Can you work these out from the model? Positions are in its coordinate system, mm. A direction names the side the tool comes from. Round coordinates to 2 decimals unless told otherwise and drop trailing zeros. Loops run counter-clockwise (first coordinate to the right, second up) from the corner with the lowest first, then second, coordinate; pieces in that order, holes last.
Autodesk Inventor part; units mm, degrees
ref_plane "YZ Plane" through (0, 0, 0) normal (1, 0, 0) x (0, 1, 0)
ref_plane "XZ Plane" through (0, 0, 0) normal (0, 1, 0) x (-1, 0, 0)
ref_plane "XY Plane" through (0, 0, 0) normal (0, 0, 1) x (1, 0, 0)
sketch "스케치1" plane through (0, 0, 0) normal (0, 0, 1) x (1, 0, 0)
  line L0 (-15, 12.75) -> (15, 12.75)
  line L1 (15, 12.75) -> (15, -12.75)
  line L2 (15, -12.75) -> (-15, -12.75)
  line L3 (-15, -12.75) -> (-15, 12.75)
  line L4 (-15, 12.75) -> (15, -12.75) construction
  line L5 (15, 12.75) -> (-15, -12.75) construction
  point P0 (0, 0)
  dimension "d0" = 30
  dimension "d1" = 25.5
extrude "돌출1" add sketch "스케치1" along normal blind 0.6
sketch "스케치2" plane through (0, 0, 0.6) normal (0, 0, 1) x (1, 0, 0)
  line L0 (-12, 12.5) -> (12, 12.5) construction
  line L1 (12, 12.5) -> (12, -12.5) construction
  line L2 (12, -12.5) -> (-12, -12.5) construction
  line L3 (-12, -12.5) -> (-12, 12.5) construction
  line L4 (-12, 12.5) -> (12, -12.5) construction
  line L5 (12, 12.5) -> (-12, -12.5) construction
  circle A0 centre (-12, 12.5) radius 1.35
  line L6 (0, 0) -> (2.9339, 0)
  line L7 (0, 0) -> (0, 3.0969)
  circle A1 centre (12, 12.5) radius 1.35
  circle A2 centre (-12, -12.5) radius 1.35
  circle A3 centre (12, -12.5) radius 1.35
  dimension "d4" = 24
  dimension "d5" = 25
  dimension "d6" = 2.7
extrude "돌출2" cut sketch "스케치2" against normal blind 0.6
sketch "스케치3" plane through (0, 0, 0.6) normal (0, 0, 1) x (1, 0, 0)
  line L0 (-6.5, 6.5) -> (6.5, 6.5)
  line L1 (6.5, 6.5) -> (6.5, -6.5)
  line L2 (6.5, -6.5) -> (-6.5, -6.5)
  line L3 (-6.5, -6.5) -> (-6.5, 6.5)
  line L4 (-6.5, 6.5) -> (6.5, -6.5) construction
  line L5 (6.5, 6.5) -> (-6.5, -6.5) construction
  circle A0 centre (8.9, 0) radius 2.1
  line L6 (8.9, 2.1) -> (6.5, 2.1)
  line L7 (8.9, -2.1) -> (6.5, -2.1)
  line L8 (0, 0) -> (0, 1.8337)
  circle A1 centre (-8.9, 0) radius 2.1
  line L9 (-8.9, 2.1) -> (-6.5, 2.1)
  line L10 (-8.9, -2.1) -> (-6.5, -2.1)
  dimension "d9" = 13
  dimension "d10" = 13
  dimension "d11" = 4.2
  dimension "d12" = 17.8
extrude "돌출3" add sketch "스케치3" along normal blind 2.7
sketch "스케치4" plane through (0, 0, 3.3) normal (0, 0, 1) x (1, 0, 0)
  circle A0 centre (0, 0) radius 4.5
  dimension "d15" = 9
extrude "돌출4" add sketch "스케치4" along normal blind 3
properties part number "카메라"
(1) If we section it at B-B, the plane x = 0: List the corners of the cut face in (y, z) for me.
Worked answers:
outline: (-12.75, 0) - (12.75, 0) - (12.75, 0.6) - (6.5, 0.6) - (6.5, 3.3) - (4.5, 3.3) - (4.5, 6.3) - (-4.5, 6.3) - (-4.5, 3.3) - (-6.5, 3.3) - (-6.5, 0.6) - (-12.75, 0.6) - close
(2) For faces 1 (the flat face through (-8, -2.1, 2)), 2 (the cylindrical face through (11, 0, 2)), 3 (the flat face through (6.5, 4, 2)), 4 (the flat face through (6.5, -4, 2)), 5 (the cylindrical face through (-0.59, -4.46, 4.78)), which set-ups out of +Z, -Z, +X, -X, +Y, -Y let a thin tool reach every point of the face, with its end or its side?
Worked answers:
face 1: +Z, -X, -Y
face 2: +Z, +X
face 3: +Z, +X, +Y
face 4: +Z, +X, -Y
face 5: +Z
(3) If we section it at D-D, the plane x = 9.25: List the corners of the cut face in (y, z) for me, then the cut area to 3 significant figures.
Worked answers:
outline: (-12.75, 0) - (12.75, 0) - (12.75, 0.6) - (2.07, 0.6) - (2.07, 3.3) - (-2.07, 3.3) - (-2.07, 0.6) - (-12.75, 0.6) - close
area: 26.5 mm2
(4) Will these pins go through, and if not, where does the flat tip stop? P1, Ø0.7, axis at x = 8, z = 2.5, coming from the -Y side; P2, Ø1, axis at x = 7.5, z = 1.5, coming from the +Y side; P3, Ø1.5, axis at y = 4.5, z = 3, coming from the -X side.
Worked answers:
P1: stops at y = -2.1
P2: stops at y = 2.1
P3: stops at x = -6.5
(5) If we mould it in two halves opening along Y, with no side actions, what happens to faces 6 (the cylindrical face through (-11, 0, 2)), 7 (the cylindrical face through (12.03, -11.15, 0.3)), 8 (the flat face through (-6.5, -4, 2))? For each: released by +Y, released by -Y, zero draft, split by the parting line, or undercut.
Worked answers:
face 6: split by the parting line
face 7: undercut
face 8: zero draft
(6) If I drill on line 1 (X direction, y = 12.5, z = 0.3); line 2 (Y direction, x = 12, z = 0.45); line 3 (Z direction, x = -11, y = -7.75), over which ranges is the centre line in solid material (lowest first)?
Worked answers:
line 1: x = -15 to -13.35, -10.65 to 10.65, 13.35 to 15
line 2: y = -11.15 to 11.15
line 3: z = 0 to 0.6
(7) If we section it at A-A, the plane z = 1: List the corners of the cut face in (x, y) for me.
Worked answers:
outline: (-8.9, -2.1) - (-6.5, -2.1) - (-6.5, -6.5) - (6.5, -6.5) - (6.5, -2.1) - (8.9, -2.1) arc R2.1 ccw to (8.9, 2.1) - (6.5, 2.1) - (6.5, 6.5) - (-6.5, 6.5) - (-6.5, 2.1) - (-8.9, 2.1) arc R2.1 ccw to start
(8) If we section it at C-C, the plane y = 5.25: List the corners of the cut face in (x, z) for me.
Worked answers:
outline: (-15, 0) - (15, 0) - (15, 0.6) - (6.5, 0.6) - (6.5, 3.3) - (-6.5, 3.3) - (-6.5, 0.6) - (-15, 0.6) - close
